Part model, mm, in its own coordinate system. A direction names the side the tool comes from. Coordinates: 2 decimals unless noted, no trailing zeros. Loops run counter-clockwise (first coordinate to the right, second up) from the corner with the lowest first, then second, coordinate; pieces in that order, holes last.
```python
from build123d import *

# Parameters (mm, degrees)
BOSS_EXTRUDE1_DEPTH      = 10
BOSS_EXTRUDE1_DEPTH_BACK = 147
SKETCH3_W                = 137
SKETCH3_H                = 550
CUT_EXTRUDE1_DEPTH       = 885
SKETCH4_W                = 137
SKETCH4_H                = 200
BOSS_EXTRUDE2_DEPTH      = 10
SKETCH5_R                = 4.5
CUT_EXTRUDE2_DEPTH       = 158
CUT_EXTRUDE3_REACH       = 82
SKETCH6_R                = 4.5
SKETCH6_R_2              = 8
CUT_EXTRUDE4_REACH       = 12
SKETCH7_R                = 4.5
SKETCH7_R_2              = 5
FILLET1_R                = 10


with BuildPart() as part:
    # Sketch1 → Boss-Extrude1 (new body, two sides)
    with BuildSketch(Plane(origin=(0, 0, 0), x_dir=(0, 0, -1), z_dir=(1, 0, 0))) as boss_extrude1_sk:
        Polygon((0, 0), (0, 750), (145, 895), (550, 895), (550, 695), (200, 695), (200, 0), align=None)
    extrude(amount=BOSS_EXTRUDE1_DEPTH)
    extrude(boss_extrude1_sk.sketch, amount=-BOSS_EXTRUDE1_DEPTH_BACK)

    # Sketch3 → Cut-Extrude1 (cut)
    with BuildSketch(Plane(origin=(0, 895, 0), x_dir=(1, 0, 0), z_dir=(0, 1, 0))):
        with Locations((-68.5, 275)):
            Rectangle(SKETCH3_W, SKETCH3_H)
    extrude(amount=-CUT_EXTRUDE1_DEPTH, mode=Mode.SUBTRACT)

    # Sketch4 → Boss-Extrude2 (add)
    with BuildSketch(Plane(origin=(0, 0, -480), x_dir=(-1, 0, 0), z_dir=(0, 0, -1))):
        with Locations((68.5, 795)):
            Rectangle(SKETCH4_W, SKETCH4_H)
    extrude(amount=-BOSS_EXTRUDE2_DEPTH)

    # Sketch5 → Cut-Extrude2 (cut, through all)
    with BuildSketch(Plane(origin=(10, 0, 0), x_dir=(0, 0, -1), z_dir=(1, 0, 0))):
        with Locations((538.25, 747.2)):
            Circle(SKETCH5_R)
        with Locations((538.25, 793.7)):
            Circle(SKETCH5_R)
        with Locations((491.75, 747.2)):
            Circle(SKETCH5_R)
        with Locations((491.75, 793.7)):
            Circle(SKETCH5_R)
    extrude(amount=-CUT_EXTRUDE2_DEPTH, mode=Mode.SUBTRACT)

    # Sketch6 → Cut-Extrude3 (cut, up to next)
    with BuildSketch(Plane.XY.offset(-470), mode=Mode.PRIVATE) as cut_extrude3_sk1:
        with Locations((-111, 747.2)):
            Circle(SKETCH6_R)
    cut_extrude3_tool1 = extrude(cut_extrude3_sk1.sketch, amount=-CUT_EXTRUDE3_REACH, mode=Mode.PRIVATE) & part.part
    add(cut_extrude3_tool1.solids().sort_by_distance((-111, 747.2, -470))[0], mode=Mode.SUBTRACT)
    # Sketch6 → Cut-Extrude3 (cut, up to next)
    with BuildSketch(Plane.XY.offset(-470), mode=Mode.PRIVATE) as cut_extrude3_sk2:
        with Locations((-26, 747.2)):
            Circle(SKETCH6_R)
    cut_extrude3_tool2 = extrude(cut_extrude3_sk2.sketch, amount=-CUT_EXTRUDE3_REACH, mode=Mode.PRIVATE) & part.part
    add(cut_extrude3_tool2.solids().sort_by_distance((-26, 747.2, -470))[0], mode=Mode.SUBTRACT)
    # Sketch6 → Cut-Extrude3 (cut, up to next)
    with BuildSketch(Plane.XY.offset(-470), mode=Mode.PRIVATE) as cut_extrude3_sk3:
        with Locations((-111, 793.7)):
            Circle(SKETCH6_R)
    cut_extrude3_tool3 = extrude(cut_extrude3_sk3.sketch, amount=-CUT_EXTRUDE3_REACH, mode=Mode.PRIVATE) & part.part
    add(cut_extrude3_tool3.solids().sort_by_distance((-111, 793.7, -470))[0], mode=Mode.SUBTRACT)
    # Sketch6 → Cut-Extrude3 (cut, up to next)
    with BuildSketch(Plane.XY.offset(-470), mode=Mode.PRIVATE) as cut_extrude3_sk4:
        with Locations((-26, 793.7)):
            Circle(SKETCH6_R)
    cut_extrude3_tool4 = extrude(cut_extrude3_sk4.sketch, amount=-CUT_EXTRUDE3_REACH, mode=Mode.PRIVATE) & part.part
    add(cut_extrude3_tool4.solids().sort_by_distance((-26, 793.7, -470))[0], mode=Mode.SUBTRACT)
    # Sketch6 → Cut-Extrude3 (cut, up to next)
    with BuildSketch(Plane.XY.offset(-470), mode=Mode.PRIVATE) as cut_extrude3_sk5:
        with Locations((-63, 788.5)):
            Circle(SKETCH6_R_2)
    cut_extrude3_tool5 = extrude(cut_extrude3_sk5.sketch, amount=-CUT_EXTRUDE3_REACH, mode=Mode.PRIVATE) & part.part
    add(cut_extrude3_tool5.solids().sort_by_distance((-63, 788.5, -470))[0], mode=Mode.SUBTRACT)

    # Sketch7 → Cut-Extrude4 (cut, up to next)
    with BuildSketch(Plane(origin=(0, 10, 0), x_dir=(1, 0, 0), z_dir=(0, 1, 0)), mode=Mode.PRIVATE) as cut_extrude4_sk1:
        with Locations((-113.5, 175)):
            Circle(SKETCH7_R)
    cut_extrude4_tool1 = extrude(cut_extrude4_sk1.sketch, amount=-CUT_EXTRUDE4_REACH, mode=Mode.PRIVATE) & part.part
    add(cut_extrude4_tool1.solids().sort_by_distance((-113.5, 10, -175))[0], mode=Mode.SUBTRACT)
    # Sketch7 → Cut-Extrude4 (cut, up to next)
    with BuildSketch(Plane(origin=(0, 10, 0), x_dir=(1, 0, 0), z_dir=(0, 1, 0)), mode=Mode.PRIVATE) as cut_extrude4_sk2:
        with Locations((-23.5, 175)):
            Circle(SKETCH7_R)
    cut_extrude4_tool2 = extrude(cut_extrude4_sk2.sketch, amount=-CUT_EXTRUDE4_REACH, mode=Mode.PRIVATE) & part.part
    add(cut_extrude4_tool2.solids().sort_by_distance((-23.5, 10, -175))[0], mode=Mode.SUBTRACT)
    # Sketch7 → Cut-Extrude4 (cut, up to next)
    with BuildSketch(Plane(origin=(0, 10, 0), x_dir=(1, 0, 0), z_dir=(0, 1, 0)), mode=Mode.PRIVATE) as cut_extrude4_sk3:
        with Locations((-23.5, 25)):
            Circle(SKETCH7_R)
    cut_extrude4_tool3 = extrude(cut_extrude4_sk3.sketch, amount=-CUT_EXTRUDE4_REACH, mode=Mode.PRIVATE) & part.part
    add(cut_extrude4_tool3.solids().sort_by_distance((-23.5, 10, -25))[0], mode=Mode.SUBTRACT)
    # Sketch7 → Cut-Extrude4 (cut, up to next)
    with BuildSketch(Plane(origin=(0, 10, 0), x_dir=(1, 0, 0), z_dir=(0, 1, 0)), mode=Mode.PRIVATE) as cut_extrude4_sk4:
        with Locations((-113.5, 25)):
            Circle(SKETCH7_R)
    cut_extrude4_tool4 = extrude(cut_extrude4_sk4.sketch, amount=-CUT_EXTRUDE4_REACH, mode=Mode.PRIVATE) & part.part
    add(cut_extrude4_tool4.solids().sort_by_distance((-113.5, 10, -25))[0], mode=Mode.SUBTRACT)
    # Sketch7 → Cut-Extrude4 (cut, up to next)
    with BuildSketch(Plane(origin=(0, 10, 0), x_dir=(1, 0, 0), z_dir=(0, 1, 0)), mode=Mode.PRIVATE) as cut_extrude4_sk5:
        with Locations((-113.5, 155)):
            Circle(SKETCH7_R_2)
    cut_extrude4_tool5 = extrude(cut_extrude4_sk5.sketch, amount=-CUT_EXTRUDE4_REACH, mode=Mode.PRIVATE) & part.part
    add(cut_extrude4_tool5.solids().sort_by_distance((-113.5, 10, -155))[0], mode=Mode.SUBTRACT)
    # Sketch7 → Cut-Extrude4 (cut, up to next)
    with BuildSketch(Plane(origin=(0, 10, 0), x_dir=(1, 0, 0), z_dir=(0, 1, 0)), mode=Mode.PRIVATE) as cut_extrude4_sk6:
        with Locations((-23.5, 45)):
            Circle(SKETCH7_R_2)
    cut_extrude4_tool6 = extrude(cut_extrude4_sk6.sketch, amount=-CUT_EXTRUDE4_REACH, mode=Mode.PRIVATE) & part.part
    add(cut_extrude4_tool6.solids().sort_by_distance((-23.5, 10, -45))[0], mode=Mode.SUBTRACT)

    # Fillet1
    fillet1_edges = [part.edges().sort_by_distance(p)[0] for p in [
        (-142, 695, -200),
        (5, 695, -200),
    ]]
    fillet(fillet1_edges, radius=FILLET1_R)


solid = part.part
```
Q1. Mould opens along Y. For faces 5 (the flat face through (5, 821, -71)), 6 (the cylindrical face through (-59.31, 781.4, -474.93)), 7 (the flat face through (-68, 796, -480)), 8 (the flat face through (-67, 0, -101)) say: released by +Y, released by -Y, zero draft, split by the parting line, or undercut.
Q2. Saw through at B-B (z = -128). List the corners of the cut face in (x, y), plus the area to 3 significant figures.
Q3. Drop flat-ended pins along their axis: P1, Ø14.5, axis at x = -23.5, z = -175, coming from the +Y side; P2, Ø18.5, axis at x = -63, y = 788.5, coming from the +Z side; P3, Ø5, axis at x = -97, y = 762, coming from the -Z side. Give the stop position or say it passes through.
Q4. Tool access for faces 1 (the flat face through (2, 344, -200)), 2 (the flat face through (0, 796, -515)), 3 (the flat face through (0, 557, -179)), 4 (the flat face through (-68, 796, -470)): list every direction of +Z, -Z, +X, -X, +Y, -Y with a clear straight run to the whole face (end or side of a thin tool).
Q5. Probe line 1 (Y direction, x = -143, z = -538); line 2 (X direction, y = 2.75, z = -25); line 3 (Z direction, x = -23.5, y = 4). List the from-to ranges inside material, lowest first.
Q6. Saw through at A-A (y = 652). List the corners of the cut face in (x, z).
Checked values:
1. face 5: released by +Y
1. face 6: undercut
1. face 7: zero draft
1. face 8: released by -Y
2. outline: (-147, 0) - (10, 0) - (10, 878) - (0, 878) - (0, 10) - (-137, 10) - (-137, 878) - (-147, 878) - close
2. area: 18,900 mm2
3. P1: stops at y = 10
3. P2: stops at z = -470
3. P3: stops at z = -480
4. face 1: -Z, +X, -X, -Y
4. face 2: -Z, +Y, -Y
4. face 3: +Z, +Y
4. face 4: +Z, +Y, -Y
5. line 1: y = 695 to 742.71, 751.69 to 789.21, 798.19 to 895
5. line 2: x = -147 to -118, -109 to -28, -19 to 10
5. line 3: z = -200 to -179.5, -170.5 to -50, -40 to -29.5, -20.5 to 0
6. outline: (-147, -200) - (-137, -200) - (-137, 0) - (-147, 0) - close; (0, -200) - (10, -200) - (10, 0) - (0, 0) - close
